Could you check a few things on this drawing? It's one solid part, dimensions in mm from its lowest x, y, z. A direction names the side the tool comes from. Give positions to 0.01 mm unless a question says otherwise; leave off trailing zeros. Loops run counter-clockwise (first coordinate to the right, second up) from the corner with the lowest first, then second, coordinate; pieces in that order, holes last. Notation, with made-up numbers: (69.5, 1.25) - (77.5, 1.25) arc R19 cw to (77.5, 22.25) - close; hole circle Ø3 at (79.5, -8.5). An arc over 180 degrees is marked (long way). Return JSON: item names as keys, results as strings. Group by question number.
(1) I need wall thicknesses on probe 1 along Z at (x, y) = (90, 7.75); probe 2 along Z at (x, y) = (50, 5.25); probe 3 along X at (y, z) = (13.75, 44). Which ranges of each line are inside material? Lowest first, please. Write a range as [from, to].
(2) On a 3-axis mill with a long thin cutter (end or side, diameter ignored), from which of +Z, -Z, +X, -X, +Y, -Y can I reach the whole of each face in a straight line? I mean the marked faces 5, 6, 7, 8 and 9. Say none if no direction works.
(3) For P1, Ø5.5, axis at x = 54.5, y = 20, coming from the -Z side; P2, Ø9, axis at x = 44.5, y = 23, coming from the +Z side; P3, Ø8, axis at x = 82.5, y = 18, coming from the -Z side, each with a flat end and sliding along its axis, tell me the tip position at first contact or that it passes through.
(4) If we section it at C-C (y = 9.75): Please give me the cut outline in (x, z), then the cut area to 3 significant figures.
(5) If we section it at B-B (z = 50): Please give me the cut outline in (x, y).
(6) If we mould it in two halves opening along X, with no side actions, what happens to the marked faces 1, 2, 3 and 4? For each: released by +X, released by -X, zero draft, split by the parting line, or undercut.
(7) If we section it at A-A (x = 50): Please give me the cut outline in (y, z), then the cut area to 3 significant figures.
(8) If we section it at D-D (x = 10): Please give me the cut outline in (y, z), then the cut area to 3 significant figures.
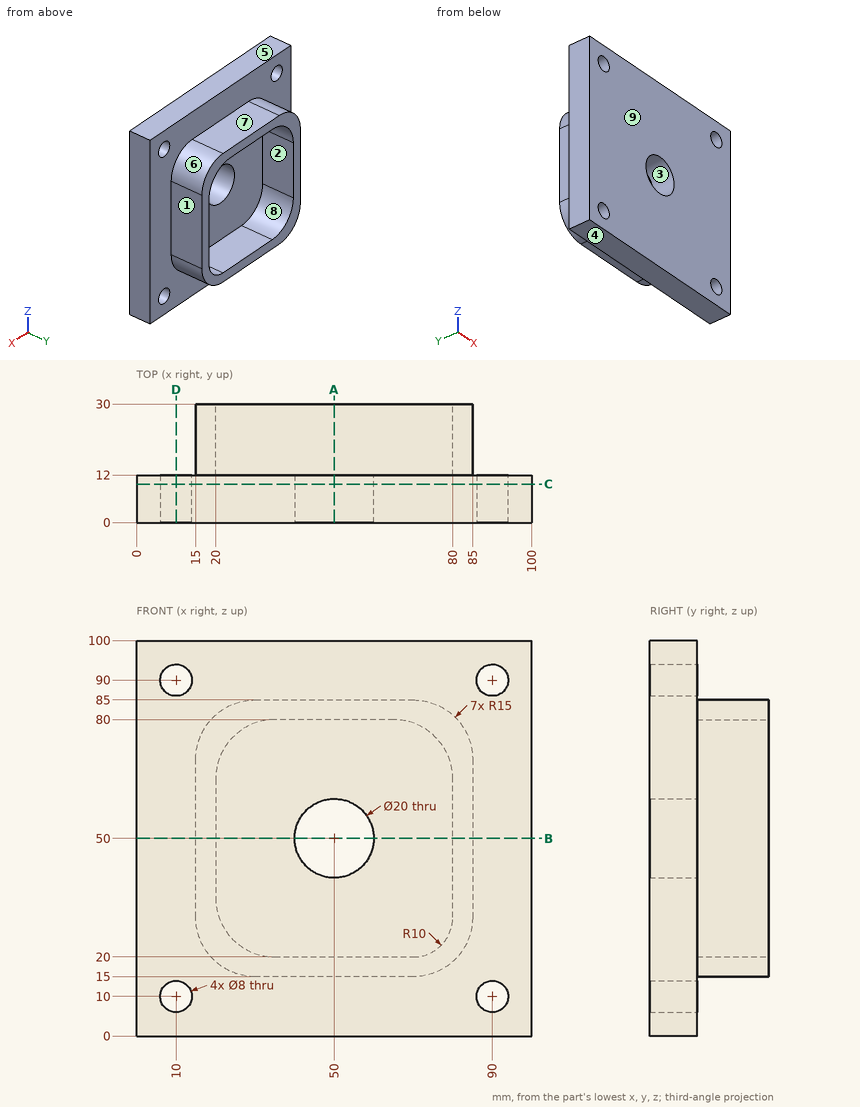
Values:
{
 "1": {"probe 1": "[0, 6], [14, 86], [94, 100]", "probe 2": "[0, 40], [60, 100]", "probe 3": "[15, 20], [80, 85]"},
 "2": {"face 5": "+Z, +X, -X, +Y, -Y", "face 6": "+Z, +X, +Y", "face 7": "+Z, +X, -X, +Y", "face 8": "+Y", "face 9": "+Z, -Z, +X, -X, -Y"},
 "3": {"P1": "z = 15", "P2": "z = 85", "P3": "z = 17.64"},
 "4": {"outline": "(0, 0) - (100, 0) - (100, 100) - (0, 100) - close; hole circle Ø8 at (10, 10); hole circle Ø8 at (10, 90); hole circle Ø20 at (50, 50); hole circle Ø8 at (90, 10); hole circle Ø8 at (90, 90)", "area": "9,480 mm2"},
 "5": {"outline": "(0, 0) - (40, 0) - (40, 12) - (20, 12) - (20, 30) - (15, 30) - (15, 12) - (0, 12) - close; (60, 0) - (100, 0) - (100, 12) - (85, 12) - (85, 30) - (80, 30) - (80, 12) - (60, 12) - close"},
 "6": {"face 1": "released by +X", "face 2": "undercut", "face 3": "undercut", "face 4": "zero draft"},
 "7": {"outline": "(0, 0) - (12, 0) - (12, 15) - (30, 15) - (30, 20) - (12, 20) - (12, 40) - (0, 40) - close; (0, 60) - (12, 60) - (12, 80) - (30, 80) - (30, 85) - (12, 85) - (12, 100) - (0, 100) - close", "area": "1,140 mm2"},
 "8": {"outline": "(0, 0) - (12, 0) - (12, 6) - (0, 6) - close; (0, 14) - (12, 14) - (12, 86) - (0, 86) - close; (0, 94) - (12, 94) - (12, 100) - (0, 100) - close", "area": "1,010 mm2"}
}
